Work out the finished part from the listing and answer in its coordinate system (mm). A direction names the side the tool comes from. Round coordinates to 2 decimals unless told otherwise and drop trailing zeros. Loops run counter-clockwise (first coordinate to the right, second up) from the corner with the lowest first, then second, coordinate; pieces in that order, holes last. Notation, with made-up numbers: (13, 7) - (34, 7) arc R10 cw to (34, 19) - close; hole circle Ø9 at (-25, 85.25). An arc over 180 degrees is marked (long way). Return JSON: item names as keys, results as strings.
from build123d import *

# Parameters (mm, degrees)
LED_BASE_BOSS_EXTRUDE1_DEPTH                   = 2.4
PIN_RIGHT_BOSS_EXTRUDE2_DEPTH                  = 2.2
PIN_RIGHT_SPACE_CUT_EXTRUDE1_REACH             = 11.15
SKETCH5_W                                      = 3.7
SKETCH5_H                                      = 0.7
PIN_RIGHT_SPACE_CUT_EXTRUDE1_DIRECTION_2_REACH = 11.15
SKETCH6_R                                      = 2.7
HEATSINK_BOSS_EXTRUDE3_DEPTH                   = 0.1


with BuildPart() as part:
    # Sketch1 → LED Base Boss-Extrude1 (new body)
    with BuildSketch(Plane(origin=(0, 0, 0), x_dir=(1, 0, 0), z_dir=(0, 1, 0))):
        with BuildLine():
            Line((-3.6, 1.743559577), (-3.6, -1.743559577))
            ThreePointArc((-3.6, -1.743559577), (0, -4), (3.6, -1.743559577))
            Line((3.6, -1.743559577), (3.6, 1.743559577))
            ThreePointArc((3.6, 1.743559577), (0, 4), (-3.6, 1.743559577))
        make_face()
    extrude(amount=LED_BASE_BOSS_EXTRUDE1_DEPTH)

    # Sketch3 → LED Lens Revolve2 (revolve)
    with BuildSketch(Plane.XY):
        with BuildLine():
            Line((2.6, 2.4), (0, 2.4))
            Line((0, 2.4), (0, 5.2))
            ThreePointArc((0, 5.2), (1.910497317, 4.366890366), (2.6, 2.4))
        make_face()
    revolve(axis=Axis((0, 5.2, 0), (0, -1, 0)))

    # Sketch4 → Pin Right Boss-Extrude2 (add, symmetric)
    with BuildSketch(Plane.XY):
        with BuildLine():
            Line((3.6, 1.4), (4.9, 1.4))
            ThreePointArc((4.9, 1.4), (5.006066017, 1.443933983), (5.05, 1.55))
            Line((5.05, 1.55), (5.05, 2.05))
            ThreePointArc((5.05, 2.05), (5.181801948, 2.368198052), (5.5, 2.5))
            Line((5.5, 2.5), (7.3, 2.5))
            Line((7.3, 2.5), (7.3, 2.2))
            Line((7.3, 2.2), (5.5, 2.2))
            ThreePointArc((5.5, 2.2), (5.393933983, 2.156066017), (5.35, 2.05))
            Line((5.35, 2.05), (5.35, 1.55))
            ThreePointArc((5.35, 1.55), (5.218198052, 1.231801948), (4.9, 1.1))
            Line((4.9, 1.1), (3.6, 1.1))
            Line((3.6, 1.1), (3.6, 1.4))
        make_face()
    pin_right_boss_extrude2 = extrude(amount=PIN_RIGHT_BOSS_EXTRUDE2_DEPTH, both=True)

    # Pin Right Space Cut-Extrude1: up to this face of the body (flat: up to its plane)
    pin_right_space_cut_extrude1_end = Plane(part.part.faces().sort_by_distance((6.4, 2.5, 0))[0])
    # Sketch5 → Pin Right Space Cut-Extrude1 (cut, up to the picked face)
    with BuildSketch(Plane(origin=(0, 1.4, 0), x_dir=(1, 0, 0), z_dir=(0, 1, 0)), mode=Mode.PRIVATE) as pin_right_space_cut_extrude1_sk1:
        with Locations((5.45, 0.85)):
            Rectangle(SKETCH5_W, SKETCH5_H)
    pin_right_space_cut_extrude1_tool1 = split(extrude(pin_right_space_cut_extrude1_sk1.sketch, amount=PIN_RIGHT_SPACE_CUT_EXTRUDE1_REACH, mode=Mode.PRIVATE), bisect_by=pin_right_space_cut_extrude1_end, keep=Keep.BOTH, mode=Mode.PRIVATE)
    # Sketch5 → Pin Right Space Cut-Extrude1 (cut, up to the picked face)
    with BuildSketch(Plane(origin=(0, 1.4, 0), x_dir=(1, 0, 0), z_dir=(0, 1, 0)), mode=Mode.PRIVATE) as pin_right_space_cut_extrude1_sk2:
        with Locations((5.45, -0.85)):
            Rectangle(SKETCH5_W, SKETCH5_H)
    pin_right_space_cut_extrude1_tool2 = split(extrude(pin_right_space_cut_extrude1_sk2.sketch, amount=PIN_RIGHT_SPACE_CUT_EXTRUDE1_REACH, mode=Mode.PRIVATE), bisect_by=pin_right_space_cut_extrude1_end, keep=Keep.BOTH, mode=Mode.PRIVATE)
    pin_right_space_cut_extrude1_1 = pin_right_space_cut_extrude1_tool1.solids().sort_by(Axis((5.45, 1.4, -0.85), (0, 1, 0)))[0]
    add(pin_right_space_cut_extrude1_1, mode=Mode.SUBTRACT)
    pin_right_space_cut_extrude1_2 = pin_right_space_cut_extrude1_tool2.solids().sort_by(Axis((5.45, 1.4, 0.85), (0, 1, 0)))[0]
    add(pin_right_space_cut_extrude1_2, mode=Mode.SUBTRACT)
    pin_right_space_cut_extrude1 = pin_right_space_cut_extrude1_1 + pin_right_space_cut_extrude1_2  # Pin Right Space Cut-Extrude1 as one shape, for the pattern or mirror that repeats it

    # Pin Right Space Cut-Extrude1 direction 2: up to this face of the body (flat: up to its plane)
    pin_right_space_cut_extrude1_direction_2_end = Plane(part.part.faces().sort_by_distance((4.25, 1.1, 0))[0])
    # Sketch5 → Pin Right Space Cut-Extrude1 direction 2 (cut, up to the picked face)
    with BuildSketch(Plane(origin=(0, 1.4, 0), x_dir=(1, 0, 0), z_dir=(0, 1, 0)), mode=Mode.PRIVATE) as pin_right_space_cut_extrude1_direction_2_sk1:
        with Locations((5.45, 0.85)):
            Rectangle(SKETCH5_W, SKETCH5_H)
    pin_right_space_cut_extrude1_direction_2_tool1 = split(extrude(pin_right_space_cut_extrude1_direction_2_sk1.sketch, amount=-PIN_RIGHT_SPACE_CUT_EXTRUDE1_DIRECTION_2_REACH, mode=Mode.PRIVATE), bisect_by=pin_right_space_cut_extrude1_direction_2_end, keep=Keep.BOTH, mode=Mode.PRIVATE)
    # Sketch5 → Pin Right Space Cut-Extrude1 direction 2 (cut, up to the picked face)
    with BuildSketch(Plane(origin=(0, 1.4, 0), x_dir=(1, 0, 0), z_dir=(0, 1, 0)), mode=Mode.PRIVATE) as pin_right_space_cut_extrude1_direction_2_sk2:
        with Locations((5.45, -0.85)):
            Rectangle(SKETCH5_W, SKETCH5_H)
    pin_right_space_cut_extrude1_direction_2_tool2 = split(extrude(pin_right_space_cut_extrude1_direction_2_sk2.sketch, amount=-PIN_RIGHT_SPACE_CUT_EXTRUDE1_DIRECTION_2_REACH, mode=Mode.PRIVATE), bisect_by=pin_right_space_cut_extrude1_direction_2_end, keep=Keep.BOTH, mode=Mode.PRIVATE)
    pin_right_space_cut_extrude1_direction_2_1 = pin_right_space_cut_extrude1_direction_2_tool1.solids().sort_by(Axis((5.45, 1.4, -0.85), (0, -1, 0)))[0]
    add(pin_right_space_cut_extrude1_direction_2_1, mode=Mode.SUBTRACT)
    pin_right_space_cut_extrude1_direction_2_2 = pin_right_space_cut_extrude1_direction_2_tool2.solids().sort_by(Axis((5.45, 1.4, 0.85), (0, -1, 0)))[0]
    add(pin_right_space_cut_extrude1_direction_2_2, mode=Mode.SUBTRACT)
    pin_right_space_cut_extrude1_direction_2 = pin_right_space_cut_extrude1_direction_2_1 + pin_right_space_cut_extrude1_direction_2_2  # Pin Right Space Cut-Extrude1 direction 2 as one shape, for the pattern or mirror that repeats it

    # Pin Left Mirror1: Pin Right Boss-Extrude2, Pin Right Space Cut-Extrude1, Pin Right Space Cut-Extrude1 direction 2 across plane
    add(pin_right_boss_extrude2.mirror(Plane(origin=(0, 0, 0), x_dir=(0, 0, 1), z_dir=(1, 0, 0))))
    add(pin_right_space_cut_extrude1.mirror(Plane(origin=(0, 0, 0), x_dir=(0, 0, 1), z_dir=(1, 0, 0))), mode=Mode.SUBTRACT)
    add(pin_right_space_cut_extrude1_direction_2.mirror(Plane(origin=(0, 0, 0), x_dir=(0, 0, 1), z_dir=(1, 0, 0))), mode=Mode.SUBTRACT)

    # Sketch6 → Heatsink Boss-Extrude3 (add)
    with BuildSketch(Plane.XZ):
        with Locations(Location((0, 0, 0), (0, 0, 90))):
            Circle(SKETCH6_R)
    extrude(amount=HEATSINK_BOSS_EXTRUDE3_DEPTH)


solid = part.part
1) Flat-ended cylindrical pins translate along their axes: pin 1 (0.5 mm diameter, centred on y = 1.5, z = 0, fed in from +X); pin 2 (1.5 mm diameter, centred on x = 3.5, y = 3.5, fed in from -Z); pin 3 (1.5 mm diameter, centred on x = -6, y = 2, fed in from -Z); pin 4 (0.8 mm diameter, centred on x = 6.5, z = 1.5, fed in from +Y). Find the tip coordinate at first contact, or state that the pin passes through.
Verdict:
{"pin 1": "stops at x = 5.35", "pin 2": "passes through", "pin 3": "stops at z = -2.2", "pin 4": "stops at y = 2.5"}
2) Section C-C (x = 0) is taken. Give the vertices of the cut face in (y, z).
Verdict:
{"outline": "(-0.1, -2.7) - (0, -2.7) - (0, -4) - (2.4, -4) - (2.4, -2.6) arc R2.61 ccw (long way) to (2.4, 2.6) - (2.4, 4) - (0, 4) - (0, 2.7) - (-0.1, 2.7) - close"}
3) Section A-A (x = -4) is taken. Give the vertices of the cut face in (y, z), and give its area (3 significant figures).
Verdict:
{"outline": "(1.1, -2.2) - (1.4, -2.2) - (1.4, -1.2) - (1.1, -1.2) - close; (1.1, -0.5) - (1.4, -0.5) - (1.4, 0.5) - (1.1, 0.5) - close; (1.1, 1.2) - (1.4, 1.2) - (1.4, 2.2) - (1.1, 2.2) - close", "area": "0.900 mm2"}
4) Find the intervals of material crossed by L1, parallel to Y at x = -6.25, z = 2; L2, parallel to Y at x = 3, z = -2; L3, parallel to Z at x = -2, y = 2.8, in increasing order.
Verdict:
{"L1": "y = 2.2 to 2.5", "L2": "y = 0 to 2.4", "L3": "z = -1.66 to 1.66"}
5) Section D-D (y = 3.6) is taken. Give the vertices of the cut face in (x, z).
Verdict:
{"outline": "circle Ø4.81 at (0, 0)"}
6) Determine the mould class of faces 1 (the flat face through (-4, 1.1, -2)), 2 (the flat face through (-4, 1.4, -2)) for opening direction X: pulls with the +X half, pulls with the -X half, needs draft (parallel to the pull), parting line crosses it, or undercut.
Verdict:
{"face 1": "needs draft", "face 2": "undercut"}
7) A tool of negligible diameter and unlimited length cuts with its end or side. For faces 3 (the flat face through (4, 1.4, -2)), 4 (the flat face through (-4, 1.1, 0)), 5 (the flat face through (6, 2.5, 2)), 6 (the flat face through (-6, 2.5, -2)), from which of +Z, -Z, +X, -X, +Y, -Y can it reach the whole face along a straight path? Write none if from no direction.
Verdict:
{"face 3": "+Z, -Z, +Y", "face 4": "+Z, -Z, -X, -Y", "face 5": "+Z, -Z, +X, +Y", "face 6": "+Z, -Z, -X, +Y"}
